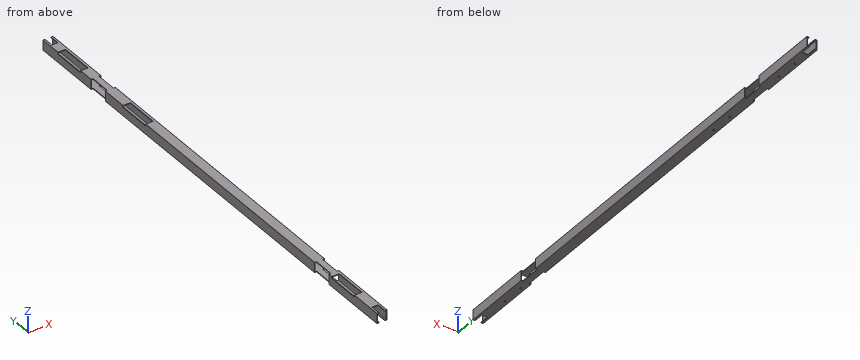
```python
from build123d import *

# Parameters (mm, degrees)
SKETCH1_W           = 17
SKETCH1_H           = 17
BOSS_EXTRUDE1_DEPTH = 975
SKETCH2_W           = 12
SKETCH2_H           = 20
CUT_EXTRUDE1_DEPTH  = 1177
SKETCH3_W           = 4
SKETCH3_H           = 42.2
CUT_EXTRUDE2_DEPTH  = 1177
SKETCH4_R           = 2.1
CUT_EXTRUDE3_DEPTH  = 10
CUT_EXTRUDE4_START  = -20
SKETCH6_W           = 4
SKETCH6_H           = 66.3
CUT_EXTRUDE4_DEPTH  = 15
LPATTERN1_COUNT     = 2
LPATTERN1_PITCH     = 190
LPATTERN2_COUNT     = 2
LPATTERN2_PITCH     = 800


with BuildPart() as part:
    # Sketch1 → Boss-Extrude1 (new body)
    with BuildSketch(Plane(origin=(0, 0, 0), x_dir=(1, 0, 0), z_dir=(0, 1, 0))):
        with BuildLine():
            Line((0.5, 0), (19.5, 0))
            ThreePointArc((19.5, 0), (19.853553391, 0.146446609), (20, 0.5))
            Line((20, 0.5), (20, 19.5))
            ThreePointArc((20, 19.5), (19.853553391, 19.853553391), (19.5, 20))
            Line((19.5, 20), (0.5, 20))
            ThreePointArc((0.5, 20), (0.146446609, 19.853553391), (0, 19.5))
            Line((0, 19.5), (0, 0.5))
            ThreePointArc((0, 0.5), (0.146446609, 0.146446609), (0.5, 0))
        make_face()
        with Locations((10, 10)):
            Rectangle(SKETCH1_W, SKETCH1_H, mode=Mode.SUBTRACT)
    extrude(amount=BOSS_EXTRUDE1_DEPTH)

    # Sketch2 → Cut-Extrude1 (cut)
    with BuildSketch(Plane.XY):
        with Locations((10, 965)):
            Rectangle(SKETCH2_W, SKETCH2_H)
    cut_extrude1 = extrude(amount=-CUT_EXTRUDE1_DEPTH, mode=Mode.SUBTRACT)

    # Sketch3 → Cut-Extrude2 (cut)
    with BuildSketch(Plane(origin=(0, 0, -20), x_dir=(-1, 0, 0), z_dir=(0, 0, -1))):
        with Locations((-2, 813.9)):
            Rectangle(SKETCH3_W, SKETCH3_H)
        with Locations((-18, 813.9)):
            Rectangle(SKETCH3_W, SKETCH3_H)
    cut_extrude2 = extrude(amount=-CUT_EXTRUDE2_DEPTH, mode=Mode.SUBTRACT)

    # Mirror1: Cut-Extrude1, Cut-Extrude2 across plane
    add(cut_extrude1.mirror(Plane.ZX.offset(487.5)), mode=Mode.SUBTRACT)
    add(cut_extrude2.mirror(Plane.ZX.offset(487.5)), mode=Mode.SUBTRACT)

    # Sketch4 → Cut-Extrude3 (cut)
    with BuildSketch(Plane.XY.offset(-20)):
        with Locations((7.75, 921.65)):
            Circle(SKETCH4_R)
        with Locations((7.75, 875.35)):
            Circle(SKETCH4_R)
    cut_extrude3 = extrude(amount=CUT_EXTRUDE3_DEPTH, mode=Mode.SUBTRACT)

    # Sketch6 → Cut-Extrude4 (cut)
    with BuildSketch(Plane(origin=(20, 0, 0), x_dir=(0, 0, -1), z_dir=(1, 0, 0)).offset(CUT_EXTRUDE4_START)):
        with Locations((2, 898.5)):
            Rectangle(SKETCH6_W, SKETCH6_H)
    cut_extrude4 = extrude(amount=CUT_EXTRUDE4_DEPTH, mode=Mode.SUBTRACT)

    # LPattern1: Cut-Extrude3, Cut-Extrude4 ×2
    with Locations(*[(0, -i * LPATTERN1_PITCH, 0) for i in range(1, LPATTERN1_COUNT)]):
        add(cut_extrude3, mode=Mode.SUBTRACT)
        add(cut_extrude4, mode=Mode.SUBTRACT)

    # LPattern2: Cut-Extrude3, Cut-Extrude4 ×2
    with Locations(*[(0, -i * LPATTERN2_PITCH, 0) for i in range(1, LPATTERN2_COUNT)]):
        add(cut_extrude3, mode=Mode.SUBTRACT)
        add(cut_extrude4, mode=Mode.SUBTRACT)


solid = part.part
```
Work out the finished part from the listing and answer in its coordinate system (mm). Coordinates: 2 decimals unless noted, no trailing zeros. Loops run counter-clockwise (first coordinate to the right, second up) from the corner with the lowest first, then second, coordinate; pieces in that order, holes last. Notation, with made-up numbers: (79, 31) - (125, 31) arc R30 ccw to (125, 60) - close; hole circle Ø11 at (49.25, 12.5). An arc over 180 degrees is marked (long way). Use a Markdown table: item, result.
Item 1: Given pin 1 Ø5.5 at (x, y) = (7.75, 921.65) entering from +Z; pin 2 Ø0.8 at (y, z) = (809, -0.5) entering from -X; pin 3 Ø1.6 at (x, y) = (1, 882) entering from +Z, each flat-ended and moving along its own axis, determine where each tip first touches the part or whether it passes through.
Evaluation:
| item | result |
|---|---|
| pin 1 | stops at z = -18.5 |
| pin 2 | stops at x = 4 |
| pin 3 | stops at z = -4 |
Item 2: Consider probe 1 along Y at (x, z) = (1, -13.5); probe 2 along X at (y, z) = (301, -9.75); probe 3 along X at (y, z) = (121.65, -19.45). Determine where each line is inside the solid, lowest interval first. Write a range as from..to.
Evaluation:
| item | result |
|---|---|
| probe 1 | y = 0..140, 182.2..792.8, 835..975 |
| probe 2 | x = 0..1.5, 18.5..20 |
| probe 3 | x = 0..5.65, 9.85..20 |
Item 3: Find section A-A, the plane z = -13. Determine the outline of the cut face in (x, y), and give its area (3 significant figures).
Evaluation:
| item | result |
|---|---|
| outline | (0, 0) - (1.5, 0) - (1.5, 140) - (0, 140) - close; (0, 182.2) - (1.5, 182.2) - (1.5, 792.8) - (0, 792.8) - close; (0, 835) - (1.5, 835) - (1.5, 975) - (0, 975) - close; (18.5, 0) - (20, 0) - (20, 140) - (18.5, 140) - close; (18.5, 182.2) - (20, 182.2) - (20, 792.8) - (18.5, 792.8) - close; (18.5, 835) - (20, 835) - (20, 975) - (18.5, 975) - close |
| area | 2,670 mm2 |
Item 4: Find section B-B, the plane y = 217. Determine the outline of the cut face in (x, z).
Evaluation:
| item | result |
|---|---|
| outline | (0, -19.5) arc R0.5 ccw to (0.5, -20) - (19.5, -20) arc R0.5 ccw to (20, -19.5) - (20, -0.5) arc R0.5 ccw to (19.5, 0) - (0.5, 0) arc R0.5 ccw to (0, -0.5) - close; hole (1.5, -18.5) - (18.5, -18.5) - (18.5, -1.5) - (1.5, -1.5) - close |
